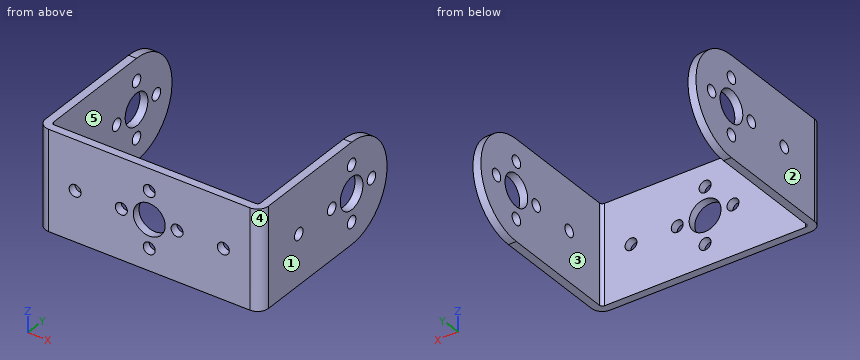
from build123d import *

# Parameters (mm, degrees)
SKETCH_1_W                       = 52
SKETCH_1_H                       = 25
SM_BASE_FLANGE_1_DEPTH           = 2
SM_EDGE_FLANGE_1_STRIP_W         = 9.4732
SM_EDGE_FLANGE_1_STRIP_H         = 2
SM_EDGE_FLANGE_1_STRIP_CUT_DEPTH = 25
SM_EDGE_FLANGE_1_DEPTH           = 25
SM_START                         = 2
SM_EDGE_FLANGE_1_FLAT_DEPTH      = 2
HOLE_WIZARD_3_0_3_1_D            = 3
HOLE_WIZARD_8_0_8_1_D            = 8
HOLE_WIZARD_3_0_3_2_D            = 3
HOLE_WIZARD_8_0_8_2_D            = 8


# Sheet-metal steps are written as plain solids
with BuildPart() as part:
    # Sketch 1 → 基体-法兰1 (new body)
    with BuildSketch(Plane(origin=(0, 0, 0), x_dir=(1, 0, 0), z_dir=(0, 1, 0))):
        Rectangle(SKETCH_1_W, SKETCH_1_H)
    extrude(amount=-SM_BASE_FLANGE_1_DEPTH)

    # 边线-法兰1 strip (across the edge) → 边线-法兰1 strip cut (cut)
    with BuildSketch(Plane(origin=(26, 0, 12.5), x_dir=(-1, 0, 0), z_dir=(0, 0, -1))):
        with Locations((-4, -1)):
            Rectangle(SM_EDGE_FLANGE_1_STRIP_W, SM_EDGE_FLANGE_1_STRIP_H)
    sm_edge_flange_1_strip_cut = extrude(amount=SM_EDGE_FLANGE_1_STRIP_CUT_DEPTH, mode=Mode.SUBTRACT)

    # 边线-法兰1 bend section (across the edge) → 边线-法兰1 (add)
    with BuildSketch(Plane(origin=(26, 0, 12.5), x_dir=(-1, 0, 0), z_dir=(0, 0, -1))):
        with BuildLine():
            Line((-2, 0.7366), (0, 0.7366))
            ThreePointArc((0, 0.7366), (0.215745145, 0.215745145), (0.7366, 0))
            Line((0.7366, 0), (0.7366, -2))
            ThreePointArc((0.7366, -2), (-1.198468417, -1.198468417), (-2, 0.7366))
        make_face()
    sm_edge_flange_1 = extrude(amount=SM_EDGE_FLANGE_1_DEPTH)

    # 边线-法兰1 profile (on flange) → 边线-法兰1 flat (add)
    with BuildSketch(Plane(origin=(26, 0, 0), x_dir=(0, 0, -1), z_dir=(1, 0, 0)).offset(SM_START)):
        with BuildLine():
            Line((-12.5, 30), (-12.5, 0.7366))
            Line((-12.5, 0.7366), (12.5, 0.7366))
            Line((12.5, 0.7366), (12.5, 30))
            ThreePointArc((12.5, 30), (0, 42.5), (-12.5, 30))
        make_face()
    sm_edge_flange_1_flat = extrude(amount=-SM_EDGE_FLANGE_1_FLAT_DEPTH)

    # 镜向1: 边线-法兰1 strip cut, 边线-法兰1, 边线-法兰1 flat across plane
    add(sm_edge_flange_1_strip_cut.mirror(Plane(origin=(0, 0, 0), x_dir=(0, 0, 1), z_dir=(1, 0, 0))), mode=Mode.SUBTRACT)
    add(sm_edge_flange_1.mirror(Plane(origin=(0, 0, 0), x_dir=(0, 0, 1), z_dir=(1, 0, 0))))
    add(sm_edge_flange_1_flat.mirror(Plane(origin=(0, 0, 0), x_dir=(0, 0, 1), z_dir=(1, 0, 0))))

    # Ø3.0 (3) 直径孔1 (through all)
    with Locations(Plane(origin=(0, -2, 0), x_dir=(-1, 0, 0), z_dir=(0, -1, 0))):
        with Locations((0, -7), (0, 7), (-7, 0), (7, 0), (18.6, 0), (-18.6, 0)):
            Hole(HOLE_WIZARD_3_0_3_1_D / 2)

    # Ø8.0 (8) 直径孔1 (through all)
    with Locations(Plane(origin=(0, -2, 0), x_dir=(-1, 0, 0), z_dir=(0, -1, 0))):
        with Locations((0, 0)):
            Hole(HOLE_WIZARD_8_0_8_1_D / 2)

    # Ø3.0 (3) 直径孔2 (through all)
    with Locations(Plane(origin=(28, 0, 0), x_dir=(0, 0, -1), z_dir=(1, 0, 0))):
        with Locations((0, 11.4), (0, 37), (7, 30), (-7, 30), (0, 23)):
            Hole(HOLE_WIZARD_3_0_3_2_D / 2)

    # Ø8.0 (8) 直径孔2 (through all)
    with Locations(Plane(origin=(28, 0, 0), x_dir=(0, 0, -1), z_dir=(1, 0, 0))):
        with Locations((0, 30)):
            Hole(HOLE_WIZARD_8_0_8_2_D / 2)


solid = part.part
Verification items for the finished model (mm, model axes). Face numbers are marked on the shaded views. A direction names the side the tool comes from. Round coordinates to 2 decimals unless told otherwise and drop trailing zeros. Loops run counter-clockwise (first coordinate to the right, second up) from the corner with the lowest first, then second, coordinate; pieces in that order, holes last. Notation, with made-up numbers: (14.5, -15) - (29.5, -15) arc R13 cw to (29.5, -9) - close; hole circle Ø6 at (13, -37). An arc over 180 degrees is marked (long way). Use a Markdown table: item, result. Add a question column.
1. Section check A-A, the plane x = 0. Record the boundary of the cut face in (y, z), plus the area to 3 significant figures.
2. Access from +Z, -Z, +X, -X, +Y, -Y to the whole of each face (thin tool, end or side, straight path). Record for the marked faces 4 and 5.
3. Gauge pin test, flat end, axial feed: pin 1 (5 mm diameter, centred on x = -7, z = 0, fed in from +Y). Record the tip position at first contact, or that the pin passes through.
4. Section check D-D, the plane z = 7.75. Record the boundary of the cut face in (x, y).
5. Section check C-C, the plane x = -7. Record the boundary of the cut face in (y, z), plus the area to 3 significant figures.
6. Section check B-B, the plane y = 15.5. Record the boundary of the cut face in (x, z), plus the area to 3 significant figures.
7. Thickness scan on probe 1 along Z at (x, y) = (0, -1.25); probe 2 along X at (y, z) = (14, 0.25); probe 3 along Y at (x, z) = (-18, -2.5). Record the ranges inside material, lowest first. Write a range as [from, to].
8. Release check for a two-part mould opening along X. For the marked faces 1, 2 and 3 record: released by +X, released by -X, zero draft, split by the parting line, or undercut.
Checks:
| question | item | result |
|---|---|---|
| 1 | outline | (-2, -12.5) - (0, -12.5) - (0, -8.5) - (-2, -8.5) - close; (-2, -5.5) - (0, -5.5) - (0, -4) - (-2, -4) - close; (-2, 4) - (0, 4) - (0, 5.5) - (-2, 5.5) - close; (-2, 8.5) - (0, 8.5) - (0, 12.5) - (-2, 12.5) - close |
| 1 | area | 22.0 mm^2 |
| 2 | face 4 | +Z, -Z, +X, -Y |
| 2 | face 5 | +Z, -Z, +Y |
| 3 | pin 1 | stops at y = 0 |
| 4 | outline | (-28, 0.74) arc R2.74 ccw to (-25.26, -2) - (-1.3, -2) - (-1.3, 0) - (-25.26, 0) arc R0.74 cw to (-26, 0.74) - (-26, 28.7) - (-28, 28.7) - close; (-28, 31.3) - (-26, 31.3) - (-26, 39.81) - (-28, 39.81) - close; (1.3, -2) - (25.26, -2) arc R2.74 ccw to (28, 0.74) - (28, 28.7) - (26, 28.7) - (26, 0.74) arc R0.74 cw to (25.26, 0) - (1.3, 0) - close; (26, 31.3) - (28, 31.3) - (28, 39.81) - (26, 39.81) - close |
| 5 | outline | (-2, -12.5) - (0, -12.5) - (0, -1.5) - (-2, -1.5) - close; (-2, 1.5) - (0, 1.5) - (0, 12.5) - (-2, 12.5) - close |
| 5 | area | 44.0 mm^2 |
| 6 | outline | (-28, -12.5) - (-26, -12.5) - (-26, 12.5) - (-28, 12.5) - close; (26, -12.5) - (28, -12.5) - (28, 12.5) - (26, 12.5) - close |
| 6 | area | 100 mm^2 |
| 7 | probe 1 | z = [-12.5, -8.5], [-5.5, -4], [4, 5.5], [8.5, 12.5] |
| 7 | probe 2 | x = [-28, -26], [26, 28] |
| 7 | probe 3 | y = [-2, 0] |
| 8 | face 1 | released by +X |
| 8 | face 2 | released by -X |
| 8 | face 3 | undercut |
